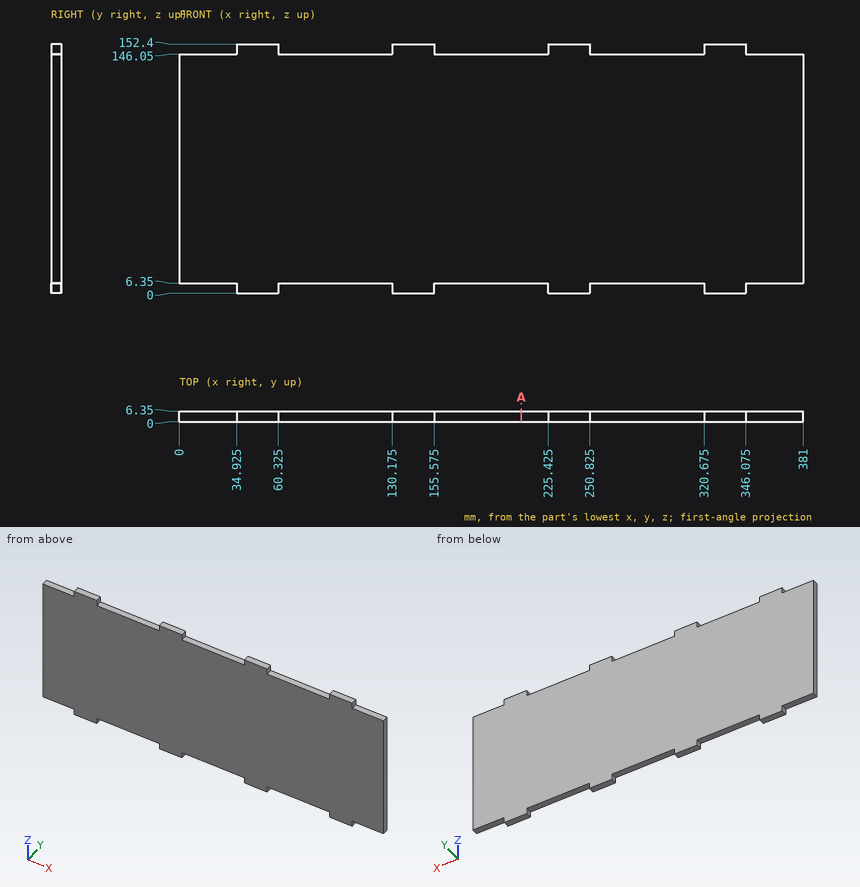
Geometry check sheet. Reference: drawing and pictorial views, mm from the part's lowest x, y, z. Round coordinates to 2 decimals unless told otherwise and drop trailing zeros. Order: outer loops, then holes, each group sorted by start corner. A loop starts at its lowest first (then second) coordinate and runs counter-clockwise, first axis right, second up. Notation, with made-up numbers: M 73,11.25 L 80,11.25 A14 ccw 80,21.25 Z; hole C -25,22 d1. An arc over 180 degrees is marked long. Answer in a Markdown table with one row per item.
(1) Go/stop test with flat-tipped pins: P1, Ø1.9, axis at y = 3, z = 149.5, coming from the -X side (3 decimals); P2, Ø3, axis at y = 3, z = 148, coming from the +X side (3 decimals); P3, Ø1.5, axis at x = 103.5, y = 3, coming from the +Z side. Record where each tip stops, or that it passes through.
Responses:
| item | result |
|---|---|
| P1 | stops at x = 34.925 |
| P2 | stops at x = 346.075 |
| P3 | stops at z = 146.05 |
(2) Sectioned sample at A-A, the plane x = 209. Record the cut outline in (y, z), and give its area (3 significant figures).
Responses:
| item | result |
|---|---|
| outline | M 0,6.35 L 6.35,6.35 L 6.35,146.05 L 0,146.05 Z |
| area | 887 mm² |
(3) Scan line: probe 1 along Z at (x, y) = (364.5, 5). Record every from-to range of solid material in increasing order. Write a range as from..to.
Responses:
| item | result |
|---|---|
| probe 1 | z = 6.35..146.05 |
